The model under review builds one solid part; all positions refer to its coordinate system, in mm. Give positions to 0.01 mm unless a question says otherwise; leave off trailing zeros. Write each loop counter-clockwise with the first axis right and the second up, starting at its lowest first coordinate (ties: lowest second). Pieces come first, ordered by that corner, then holes. Notation, with made-up numbers: (43, -37) -> (77, -37) arc R15 ccw to (77, -33) -> close; hole circle Ø11 at (-20.5, 15). An arc over 180 degrees is marked (long way). Use CSV: the item, a comma, the result in double quotes.
Autodesk Fusion 360 part; units mm, degrees
sketch "Sketch3" plane through (0, 0, 0) normal (0, 0, 1) x (1, 0, 0)
  line L0 (0, 10) -> (0, 45)
  line L1 (10, 55) -> (31.3603, 55)
  line L2 (52.8119, 0) -> (10, 0)
  line L3 (62.8119, 27) -> (52.8119, 27) construction
  line L4 (62.8119, 27) -> (62.8119, 10)
  line L5 (37.7882, 52.6604) -> (59.2397, 34.6604)
  arc A0 (62.8119, 27) -> (59.2397, 34.6604) centre (52.8119, 27) ccw
  arc A1 (37.7882, 52.6604) -> (31.3603, 55) centre (31.3603, 45) ccw
  arc A2 (10, 55) -> (0, 45) centre (10, 45) ccw
  arc A3 (52.8119, 0) -> (62.8119, 10) centre (52.8119, 10) ccw
  arc A4 (0, 10) -> (10, 0) centre (10, 10) ccw
  line L6 (0, 27) -> (28, 27) construction
  line L7 (0, 40) -> (41, 40) construction
  circle A5 centre (41, 40) radius 5
  circle A6 centre (10, 10) radius 3
  circle A7 centre (21, 10) radius 3
  circle A8 centre (10, 21) radius 3
  line L8 (7, 21) -> (7, 10)
  line L9 (10, 7) -> (21, 7)
  arc A9 (13, 21) -> (21, 13) centre (21, 21) ccw
  circle A10 centre (52.8119, 10) radius 3
  circle A11 centre (41.8119, 10) radius 3
  circle A12 centre (52.8119, 21) radius 3
  line L10 (41.8119, 7) -> (52.8119, 7)
  line L11 (55.809, 9.8683) -> (55.8119, 20.9992)
  line L12 (49.8119, 21.0011) -> (49.8119, 20.9971)
  line L13 (41.809, 13) -> (41.8129, 13)
  arc A13 (41.809, 13) -> (49.8119, 20.9971) centre (41.8119, 21) ccw
  circle A14 centre (10, 45) radius 3
  circle A15 centre (21, 45) radius 3
  circle A16 centre (10, 34) radius 3
  line L14 (7, 34) -> (7, 45)
  line L15 (10, 48) -> (21, 48)
  line L16 (21, 42) -> (21, 42)
  arc A17 (21, 42) -> (13, 34) centre (21, 34) ccw
  line L17 (41, 40) -> (41, 32) construction
  line L18 (41, 40) -> (33, 40) construction
  circle A18 centre (28, 27) radius 10.9284
  arc A19 (31.9231, 37.2) -> (36, 40) centre (33, 40) ccw
  arc A20 (41, 35) -> (38.2, 30.9231) centre (41, 32) ccw
  point P0 (0, 55)
  point P1 (60, 55)
  point P2 (35, 55)
  dimension "d35" = 55
  dimension "d36" = 60
  dimension "d37" = 25
  dimension "d39" = 10
  dimension "d40" = 28
  dimension "d41" = 20
  dimension "d42" = 140
  dimension "d43" = 10
  dimension "d44" = 10
  dimension "d45" = 10
  dimension "d46" = 10
  dimension "d51" = 28
  dimension "d52" = 28
  dimension "d53" = 41
  dimension "d54" = 15
  dimension "d55" = 10
  dimension "d56" = 6
  dimension "d57" = 6
  dimension "d58" = 6
  dimension "d60" = 55
  dimension "d62" = 11
  dimension "d63" = 11
  dimension "d64" = 8
  dimension "d65" = 6
  dimension "d66" = 6
  dimension "d67" = 6
  dimension "d68" = 8
  dimension "d69" = 11
  dimension "d70" = 11
  dimension "d71" = 6
  dimension "d72" = 6
  dimension "d73" = 6
  dimension "d74" = 11
  dimension "d75" = 11
  dimension "d76" = 8
  dimension "d79" = 8
  dimension "d80" = 8
extrude "Extrude3" add sketch "Sketch3" along normal blind 3
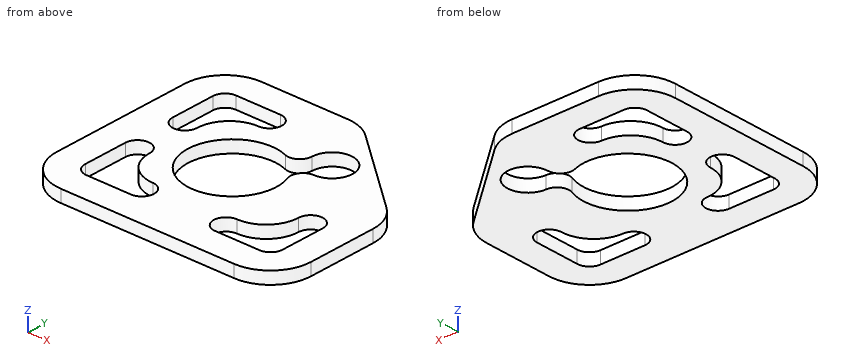
Q1. Insertion check: pin 1 (19.5 mm diameter, centred on x = 28, y = 27, fed in from -Z); pin 2 (1.5 mm diameter, centred on x = 47, z = 1, fed in from +Y). Each pin has a flat end and moves straight along its axis. Give the tip position at first contact, or say it passes through.
Derived:
pin 1,"passes through"
pin 2,"stops at y = 45.56"
Q2. Consider section D-D (z = 1.2). State how many separate pieces and enclosed holes the cut face has, then the cut area to 3 significant figures.
Derived:
separate pieces,"1"
enclosed holes,"4"
area,"2,070 mm2"
Q3. Consider section B-B (y = 23). Write out the cut boundary in (x, z).
Derived:
outline,"(0, 0) -> (7.76, 0) -> (7.76, 3) -> (0, 3) -> close; (12.24, 0) -> (17.83, 0) -> (17.83, 3) -> (12.24, 3) -> close; (38.17, 0) -> (50.58, 0) -> (50.58, 3) -> (38.17, 3) -> close; (55.05, 0) -> (62.81, 0) -> (62.81, 3) -> (55.05, 3) -> close"
Q4. Consider section A-A (x = 28). Write out the cut boundary in (y, z).
Derived:
outline,"(0, 0) -> (16.07, 0) -> (16.07, 3) -> (0, 3) -> close; (37.93, 0) -> (55, 0) -> (55, 3) -> (37.93, 3) -> close"
Q5. To check wall thickness, follow probe 1 along Y at (x, z) = (18.5, 0.6); probe 2 along X at (y, z) = (38.5, 0.65); probe 3 along Y at (x, z) = (41, 1.05). State the ranges of each line that lie inside material, in increasing order.
Derived:
probe 1,"y = 0 to 7, 13.4 to 21.6, 32.4 to 41.6, 48 to 55"
probe 2,"x = 0 to 7, 14.39 to 35.6, 45.77 to 54.66"
probe 3,"y = 0 to 7.11, 12.89 to 35, 45 to 49.97"
Q6. Consider section C-C (y = 44). Write out the cut boundary in (x, z), then the cut area to 3 significant figures.
Derived:
outline,"(0, 0) -> (7, 0) -> (7, 3) -> (0, 3) -> close; (23.83, 0) -> (38, 0) -> (38, 3) -> (23.83, 3) -> close; (44, 0) -> (48.11, 0) -> (48.11, 3) -> (44, 3) -> close"
area,"75.8 mm2"
